Here's the drawing with two shaded views (mm, measured from the low corner). I have some questions. A direction names the side the tool comes from. Coordinates: 2 decimals unless noted, no trailing zeros. Write each loop counter-clockwise with the first axis right and the second up, starting at its lowest first coordinate (ties: lowest second). Pieces come first, ordered by that corner, then holes. Notation, with made-up numbers: (11, 80) -> (35, 80) arc R17 cw to (35, 109) -> close; hole circle Ø5 at (36, -35.5). An arc over 180 degrees is marked (long way). Use one line per item in the form item = value.
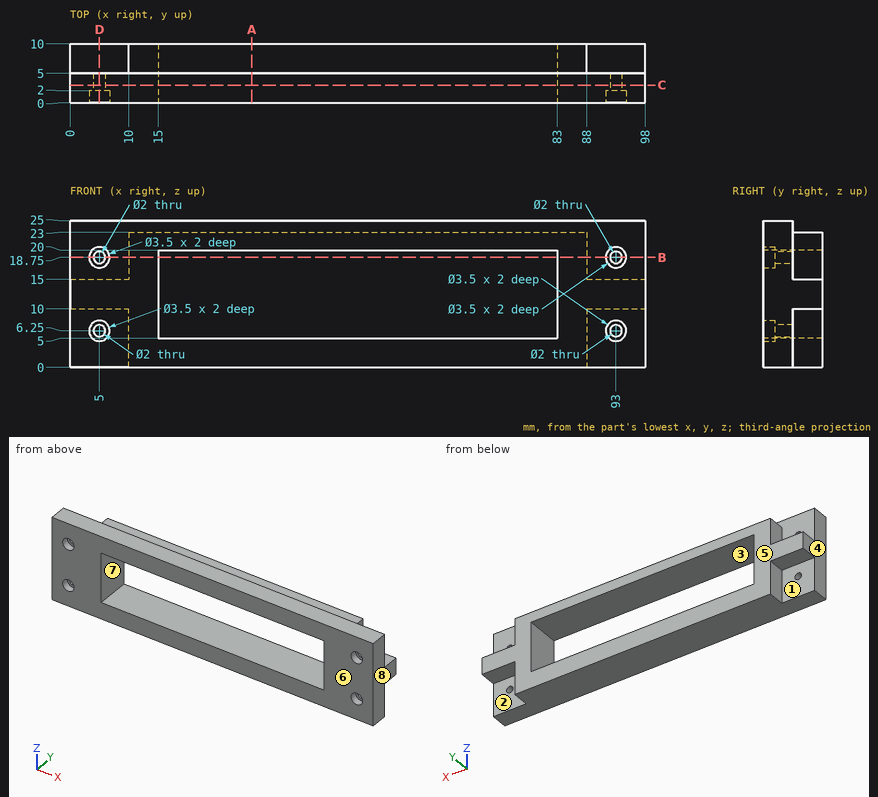
Q1. Thinking about a two-plate mould opening in X: for the marked faces 6, 7 and 8, which applies, released by +X, released by -X, zero draft, split by the parting line, or undercut?
Return value:
face_6 = zero draft
face_7 = undercut
face_8 = released by +X
Q2. Suppose I cut it at A-A (x = 31). Write out the boundary of the cut face in (y, z).
Return value:
outline = (0, 0) -> (10, 0) -> (10, 5) -> (0, 5) -> close; (0, 20) -> (10, 20) -> (10, 23) -> (5, 23) -> (5, 25) -> (0, 25) -> close
Q3. Suppose I cut it at C-C (y = 3). Write out the boundary of the cut face in (x, z).
Return value:
outline = (0, 0) -> (98, 0) -> (98, 25) -> (0, 25) -> close; hole circle Ø2 at (5, 6.25); hole circle Ø2 at (5, 18.75); hole (15, 5) -> (83, 5) -> (83, 20) -> (15, 20) -> close; hole circle Ø2 at (93, 6.25); hole circle Ø2 at (93, 18.75)
Q4. Suppose I cut it at D-D (x = 5). Write out the boundary of the cut face in (y, z).
Return value:
outline = (0, 0) -> (5, 0) -> (5, 5.25) -> (2, 5.25) -> (2, 4.5) -> (0, 4.5) -> close; (0, 8) -> (2, 8) -> (2, 7.25) -> (5, 7.25) -> (5, 10) -> (10, 10) -> (10, 15) -> (5, 15) -> (5, 17.75) -> (2, 17.75) -> (2, 17) -> (0, 17) -> close; (0, 20.5) -> (2, 20.5) -> (2, 19.75) -> (5, 19.75) -> (5, 25) -> (0, 25) -> close
Q5. If I drill on line 1 (Z direction, x = 93, y = 2.6); line 2 (X direction, y = 4.25, z = 6.25); line 3 (Z direction, x = 93, y = 1.2), over which ranges is the centre line in solid material (lowest first)? Write a range as from..to.
Return value:
line_1 = 0..5.25, 7.25..17.75, 19.75..25
line_2 = 0..4, 6..15, 83..92, 94..98
line_3 = 0..4.5, 8..17, 20.5..25
Q6. For the marked faces 1, 2, 3, 4 and 5, which set-ups out of +Z, -Z, +X, -X, +Y, -Y let a thin tool reach every point of the face, with its end or its side?
Return value:
face_1 = -Z, -X, +Y
face_2 = -Z, +X, +Y
face_3 = +Y, -Y
face_4 = +Z, -Z, -X, +Y, -Y
face_5 = +Z, -Z, +X, -X, +Y
Q7. Will these pins go through, and if not, where does the flat tip stop? pin 1 (11 mm diameter, centred on x = 26, z = 18, fed in from +Y); pin 2 (2.5 mm diameter, centred on x = 6.5, y = 7, fed in from -Z); pin 3 (1.5 mm diameter, centred on y = 7, z = 6.5, fed in from +X); pin 4 (5 mm diameter, centred on x = 79, z = 10, fed in from +Y).
Return value:
pin_1 = 10
pin_2 = 10
pin_3 = 88
pin_4 = through
Q8. Suppose I cut it at B-B (z = 18.75). Write out the boundary of the cut face in (x, y), then the cut area to 3 significant figures.
Return value:
outline = (0, 0) -> (3.25, 0) -> (3.25, 2) -> (4, 2) -> (4, 5) -> (0, 5) -> close; (6, 2) -> (6.75, 2) -> (6.75, 0) -> (15, 0) -> (15, 10) -> (10, 10) -> (10, 5) -> (6, 5) -> close; (83, 0) -> (91.25, 0) -> (91.25, 2) -> (92, 2) -> (92, 5) -> (88, 5) -> (88, 10) -> (83, 10) -> close; (94, 2) -> (94.75, 2) -> (94.75, 0) -> (98, 0) -> (98, 5) -> (94, 5) -> close
area = 174 mm2
